from build123d import *

# Parameters (mm, degrees)
SKETCH_1_R      = 24
SKETCH_1_R_2    = 3
SKETCH_1_R_3    = 1.5
EXTRUDE_1_DEPTH = 2
FILLET_1_R      = 1.5


with BuildPart() as part:
    # 草图1 → 凸台-拉伸1 (new body)
    with BuildSketch(Plane.XY):
        Circle(SKETCH_1_R)
        Circle(SKETCH_1_R_2, mode=Mode.SUBTRACT)
        with Locations((-7.368432559, 4.254166522)):
            Circle(SKETCH_1_R_3, mode=Mode.SUBTRACT)
        with Locations((7.368432559, 4.254166522)):
            Circle(SKETCH_1_R_3, mode=Mode.SUBTRACT)
        with Locations((0, -8.508333043)):
            Circle(SKETCH_1_R_3, mode=Mode.SUBTRACT)
        with BuildLine():
            Line((8.034845121, 9.575555539), (12.212964584, 14.554844419))
            ThreePointArc((12.212964584, 14.554844419), (0, 19), (-12.212964584, 14.554844419))
            Line((-12.212964584, 14.554844419), (-8.034845121, 9.575555539))
            ThreePointArc((-8.034845121, 9.575555539), (0, 12.5), (8.034845121, 9.575555539))
        make_face(mode=Mode.SUBTRACT)
        with BuildLine():
            Line((12.310096913, 2.170602221), (18.711347307, 3.299315376))
            ThreePointArc((18.711347307, 3.299315376), (16.454482672, -9.5), (6.498382723, -17.854159795))
            Line((6.498382723, -17.854159795), (4.275251792, -11.74615776))
            ThreePointArc((4.275251792, -11.74615776), (10.825317547, -6.25), (12.310096913, 2.170602221))
        make_face(mode=Mode.SUBTRACT)
        with BuildLine():
            Line((-4.275251792, -11.74615776), (-6.498382723, -17.854159795))
            ThreePointArc((-6.498382723, -17.854159795), (-16.454482672, -9.5), (-18.711347307, 3.299315376))
            Line((-18.711347307, 3.299315376), (-12.310096913, 2.170602221))
            ThreePointArc((-12.310096913, 2.170602221), (-10.825317547, -6.25), (-4.275251792, -11.74615776))
        make_face(mode=Mode.SUBTRACT)
    extrude(amount=EXTRUDE_1_DEPTH)

    # 圆角1
    fillet_1_edges = [part.edges().sort_by_distance(p)[0] for p in [
        (-8.034845121, 9.575555539, 1),
        (8.034845121, 9.575555539, 1),
        (12.212964584, 14.554844419, 1),
        (-12.212964584, 14.554844419, 1),
        (12.310096913, 2.170602221, 1),
        (4.275251792, -11.74615776, 1),
        (6.498382723, -17.854159795, 1),
        (18.711347307, 3.299315376, 1),
        (-4.275251792, -11.74615776, 1),
        (-12.310096913, 2.170602221, 1),
        (-18.711347307, 3.299315376, 1),
        (-6.498382723, -17.854159795, 1),
    ]]
    fillet(fillet_1_edges, radius=FILLET_1_R)


solid = part.part
Geometry: final body of the model. Coordinates: model frame, mm. A direction names the side the tool comes from. Coordinates: 2 decimals unless noted, no trailing zeros. Order: outer loops, then holes, each group sorted by start corner. A loop starts at its lowest first (then second) coordinate and runs counter-clockwise, first axis right, second up.
1) Draft query along Y for faces 3 (the cylindrical face through (12.778, 1.853, 1.014)), 4 (the flat face through (0, -5, 2)), 5 (the flat face through (5.37, -14.755, 0.986)). Return one class per face: released by +Y, released by -Y, zero draft, split by the parting line, or undercut.
Result sheet:
face 3: undercut
face 4: zero draft
face 5: undercut
2) First-contact query: P1, Ø10, axis at x = 14, y = 1, coming from the -Z side. Flat tip, straight axial feed; report the tip coordinate or a pass-through.
Result sheet:
P1: stops at z = 0
3) Section D-D (x = -10). Return loops of the section in (y, z), then the cut area to 3 significant figures.
Result sheet:
outline: (-21.82, 0) - (-16.16, 0) - (-16.16, 2) - (-21.82, 2) - close; (-7.5, 0) - (11.92, 0) - (11.92, 2) - (-7.5, 2) - close; (16.16, 0) - (21.82, 0) - (21.82, 2) - (16.16, 2) - close
area: 61.5 mm2
4) Section B-B (x = 0). Return loops of the section in (y, z), then the cut area to 3 significant figures.
Result sheet:
outline: (-24, 0) - (-10.01, 0) - (-10.01, 2) - (-24, 2) - close; (-7.01, 0) - (-3, 0) - (-3, 2) - (-7.01, 2) - close; (3, 0) - (12.5, 0) - (12.5, 2) - (3, 2) - close; (19, 0) - (24, 0) - (24, 2) - (19, 2) - close
area: 65.0 mm2
5) Section C-C (y = -5.5). Return loops of the section in (x, z).
Result sheet:
outline: (-23.36, 0) - (-18.19, 0) - (-18.19, 2) - (-23.36, 2) - close; (-11.22, 0) - (11.22, 0) - (11.22, 2) - (-11.22, 2) - close; (18.19, 0) - (23.36, 0) - (23.36, 2) - (18.19, 2) - close
6) Section A-A (y = 0). Return loops of the section in (x, z).
Result sheet:
outline: (-24, 0) - (-19, 0) - (-19, 2) - (-24, 2) - close; (-12.5, 0) - (-3, 0) - (-3, 2) - (-12.5, 2) - close; (3, 0) - (12.5, 0) - (12.5, 2) - (3, 2) - close; (19, 0) - (24, 0) - (24, 2) - (19, 2) - close
7) Ray query, probe 1 along Y at (x, z) = (0, 0.4); probe 2 along X at (y, z) = (-10.5, 1.05); probe 3 along X at (y, z) = (-4, 0.1). Return the intervals inside material, ascending.
Result sheet:
probe 1: y = -24 to -10.01, -7.01 to -3, 3 to 12.5, 19 to 24
probe 2: x = -21.58 to -15.84, -6.78 to 6.78, 15.84 to 21.58
probe 3: x = -23.66 to -18.57, -11.84 to 11.84, 18.57 to 23.66
8) Set-up query: faces 1 (the flat face through (0, -5, 0)), 2 (the cylindrical face through (8.024, 10.144, 1.014)). Return all of +Z, -Z, +X, -X, +Y, -Y with unobstructed straight access to the full face (end or side cutting, diameter ignored); none if empty.
Result sheet:
face 1: -Z, +X, -X, +Y, -Y
face 2: +Z, -Z
